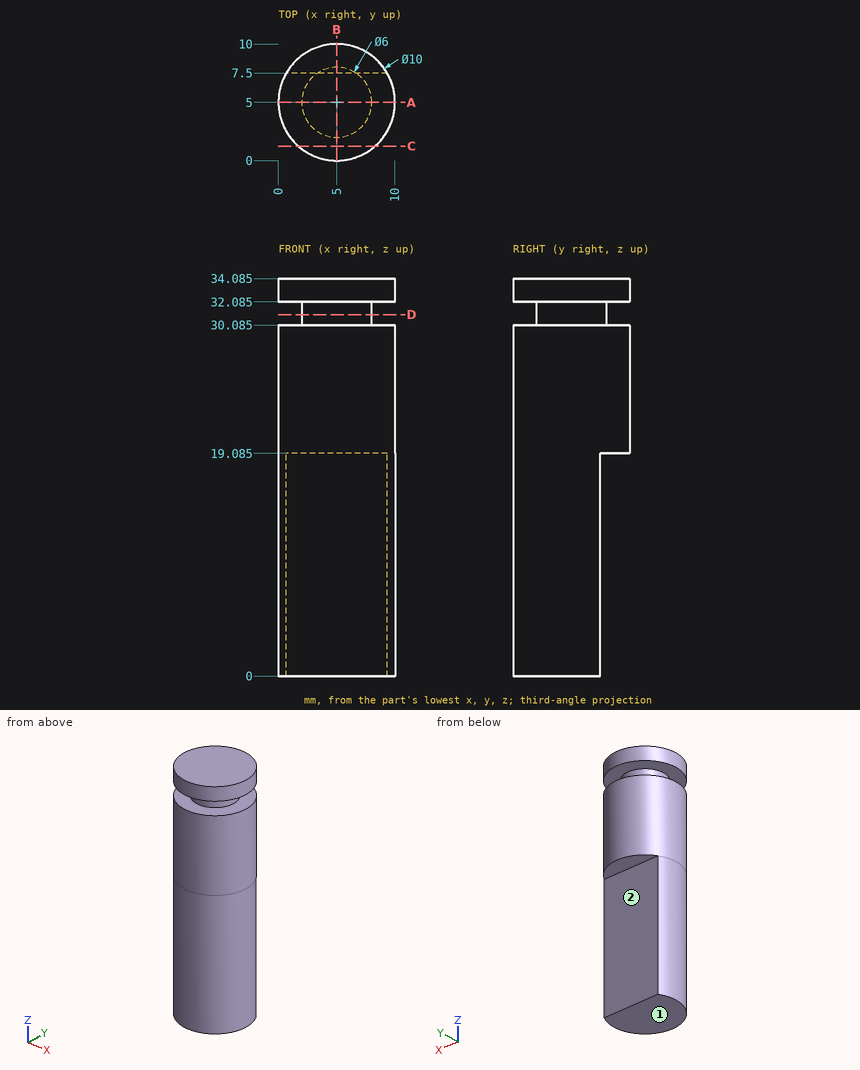
Check sheet for the drawn part. Datum: minimum x, y, z corner. Units: mm. A direction names the side the tool comes from. Round coordinates to 2 decimals unless told otherwise and drop trailing zeros. Loops run counter-clockwise (first coordinate to the right, second up) from the corner with the lowest first, then second, coordinate; pieces in that order, holes last.
Item 1: Access from +Z, -Z, +X, -X, +Y, -Y to the whole of each face (thin tool, end or side, straight path). Record for the marked faces 1 and 2.
Item 2: Thickness scan on line 1 (Z direction, x = 3.5, y = 1) (3 decimals); line 2 (Z direction, x = 4.5, y = 9.5) (3 decimals); line 3 (X direction, y = 4.75, z = 29). Record the ranges inside material, lowest first.
Item 3: Cross-section at C-C on y = 1.25. Record the boundary of the cut face in (x, z) (1 decimal).
Item 4: Cross-section at A-A on y = 5. Record the boundary of the cut face in (x, z) (3 decimals).
Item 5: Gauge pin test, flat ends, axial feed: pin 1 (0.8 mm diameter, centred on x = 5.5, y = 9, fed in from -Z) (3 decimals); pin 2 (4.5 mm diameter, centred on x = 6, z = 8, fed in from +Y); pin 3 (2 mm diameter, centred on x = 3.5, z = 7.5, fed in from -Y) (3 decimals). Record the tip position at first contact, or that the pin passes through.
Item 6: Cross-section at D-D on z = 31. Record the boundary of the cut face in (x, y), then the cut area to 3 significant figures.
Item 7: Cross-section at B-B on x = 5. Record the boundary of the cut face in (y, z) (3 decimals).
Answer sheet:
1. face 1: -Z, +X, -X, +Y, -Y
1. face 2: -Z, +X, -X, +Y
2. line 1: z = 0 to 30.085, 32.085 to 34.085
2. line 2: z = 19.085 to 30.085, 32.085 to 34.085
2. line 3: x = 0.01 to 9.99
3. outline: (1.7, 0) - (8.3, 0) - (8.3, 30.1) - (1.7, 30.1) - close; (1.7, 32.1) - (8.3, 32.1) - (8.3, 34.1) - (1.7, 34.1) - close
4. outline: (0, 0) - (10, 0) - (10, 30.085) - (8, 30.085) - (8, 32.085) - (10, 32.085) - (10, 34.085) - (0, 34.085) - (0, 32.085) - (2, 32.085) - (2, 30.085) - (0, 30.085) - close
5. pin 1: stops at z = 19.085
5. pin 2: stops at y = 7.5
5. pin 3: stops at y = 0.025
6. outline: circle Ø6 at (5, 5)
6. area: 28.3 mm2
7. outline: (0, 0) - (7.5, 0) - (7.5, 19.085) - (10, 19.085) - (10, 30.085) - (8, 30.085) - (8, 32.085) - (10, 32.085) - (10, 34.085) - (0, 34.085) - (0, 32.085) - (2, 32.085) - (2, 30.085) - (0, 30.085) - close
